Could you check a few things on this model? Use its own coordinates, in mm. Face numbers are marked on the shaded views. A direction names the side the tool comes from. Round coordinates to 2 decimals unless told otherwise and drop trailing zeros. Write each loop counter-clockwise with the first axis right and the second up, starting at its lowest first coordinate (ties: lowest second). Pieces come first, ordered by that corner, then holes. Notation, with made-up numbers: (14, 84) - (23, 84) arc R32 cw to (23, 121) - close; hole circle Ø6 at (52.25, 82.25). An arc over 180 degrees is marked (long way). Put each result on its own line as item: value.
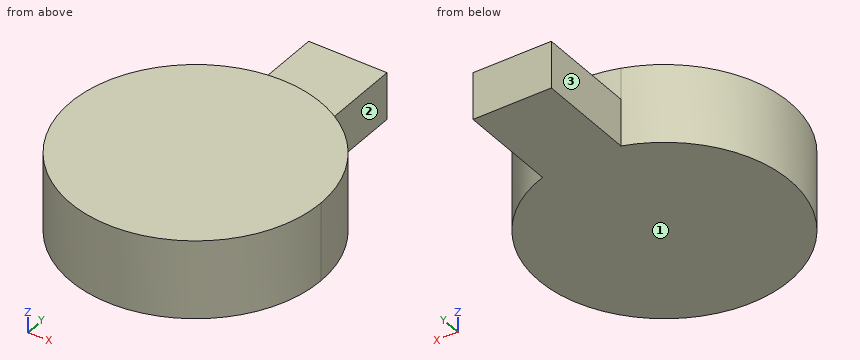
from build123d import *

# Parameters (mm, degrees)
F1_DEPTH = 3.175
F2_DEPTH = 1.905


with BuildPart() as f1:
    # F0 (on Top) → F1 (new body)
    with BuildSketch(Plane.XY):
        with BuildLine():
            ThreePointArc((-1.5875, 4.825582), (-2.978414, -4.11527), (5.08, 0))
            ThreePointArc((5.08, 0), (4.11527, 2.978414), (1.5875, 4.825582))
            ThreePointArc((1.5875, 4.825582), (0, 5.08), (-1.5875, 4.825582))
        make_face()
    extrude(amount=F1_DEPTH)

    # F0 (on Top) → F2 (join)
    with BuildSketch(Plane.XY):
        with BuildLine():
            ThreePointArc((-1.5875, 4.825582), (0, 5.08), (1.5875, 4.825582))
            Line((1.5875, 4.825582), (1.5875, 8.89))
            Line((1.5875, 8.89), (-1.5875, 8.89))
            Line((-1.5875, 8.89), (-1.5875, 4.825582))
        make_face()
    extrude(amount=F2_DEPTH)


solid = f1.part
(1) Imagine slicing it at C-C, the plane y = 4.5. List the corners of the cut face in (x, z) for me (3 decimals), then the cut area to 3 significant figures.
Values found:
outline: (-2.357, 0) - (2.357, 0) - (2.357, 3.175) - (-2.357, 3.175) - close
area: 15.0 mm^2
(2) For the marked faces 1, 2 and 3, which set-ups out of +Z, -Z, +X, -X, +Y, -Y let a thin tool reach every point of the face, with its end or its side?
Values found:
face 1: -Z, +X, -X, +Y, -Y
face 2: +Z, -Z, +X, +Y
face 3: +Z, -Z, -X, +Y
(3) Please list where these lines run through material, in increasing order: probe 1 along Y at (x, z) = (0, 2.15); probe 2 along Z at (x, y) = (0, 7) (3 decimals); probe 3 along X at (y, z) = (6.5, 0.4). Write a range as from..to.
Values found:
probe 1: y = -5.08..5.08
probe 2: z = 0..1.905
probe 3: x = -1.59..1.59
(4) Imagine slicing it at B-B, the plane z = 1.5. List the corners of the cut face in (x, y) for me, then the cut area to 3 significant figures.
Values found:
outline: (-1.59, 4.83) arc R5.08 ccw (long way) to (1.59, 4.83) - (1.59, 8.89) - (-1.59, 8.89) - close
area: 93.4 mm^2
(5) Imagine slicing it at A-A, the plane x = 0. List the corners of the cut face in (y, z) for me (3 decimals).
Values found:
outline: (-5.08, 0) - (8.89, 0) - (8.89, 1.905) - (5.08, 1.905) - (5.08, 3.175) - (-5.08, 3.175) - close
(6) I'm going to push flat-ended pins straight in: pin 1 (0.6 mm diameter, centred on y = 7.5, z = 1.5, fed in from -X); pin 2 (0.6 mm diameter, centred on y = 7.5, z = 1.5, fed in from +X). Where does each tip first touch, or does it pass through?
Values found:
pin 1: stops at x = -1.59
pin 2: stops at x = 1.59
